Part model, mm, in its own coordinate system. A direction names the side the tool comes from. Give positions to 0.01 mm unless a question says otherwise; leave off trailing zeros. Loops run counter-clockwise (first coordinate to the right, second up) from the corner with the lowest first, then second, coordinate; pieces in that order, holes last. Notation, with made-up numbers: M -17.5,58.25 L 31.5,58.25 A15 cw 31.5,68.25 Z; hole C -33,-24.75 d2. An arc over 180 degrees is marked long. Put each result on its own line as item: value. Start each with the question number.
Autodesk Inventor part; units mm, degrees
ref_plane "YZ Plane" through (0, 0, 0) normal (1, 0, 0) x (0, 1, 0)
ref_plane "XZ Plane" through (0, 0, 0) normal (0, 1, 0) x (-1, 0, 0)
ref_plane "XY Plane" through (0, 0, 0) normal (0, 0, 1) x (1, 0, 0)
sketch "Sketch1" plane through (0, 0, 0) normal (0, 0, 1) x (1, 0, 0)
  line L0 (-28.08, -48.025) -> (28.08, -48.025)
  line L1 (28.08, -48.025) -> (28.08, 48.025)
  line L2 (28.08, 48.025) -> (-28.08, 48.025)
  line L3 (-28.08, 48.025) -> (-28.08, -48.025)
  line L4 (-28.08, -48.025) -> (28.08, 48.025) construction
  line L5 (28.08, -48.025) -> (-28.08, 48.025) construction
  point P0 (0, 0)
  dimension "Length" = 56.16
  dimension "Height" = 96.05
extrude "BasicShape" add sketch "Sketch1" along normal blind 5
sketch "KeypadDimensions" plane through (0, 0, 5) normal (0, 0, 1) x (1, 0, 0)
  line L0 (-28.08, -48.025) -> (28.08, -48.025) construction
  line L1 (28.08, -48.025) -> (3.93, -48.025) construction
  line L2 (3.93, -48.025) -> (3.93, 0) construction
  line L3 (3.93, 0) -> (28.08, 0) construction
  line L4 (28.08, 0) -> (28.08, -48.025) construction
  line L5 (-20.22, -40.2) -> (28.08, -40.2)
  line L6 (28.08, -40.2) -> (28.08, 40.2)
  line L7 (28.08, 40.2) -> (-20.22, 40.2)
  line L8 (-20.22, 40.2) -> (-20.22, -40.2)
  line L9 (-20.22, -40.2) -> (28.08, 40.2) construction
  line L10 (28.08, -40.2) -> (-20.22, 40.2) construction
  point P0 (0, 0)
  dimension "d4" = 24.15
  dimension "d5" = 48.025
  dimension "KeypadLength" = 48.3
  dimension "KeypadHeight" = 80.4
extrude "KeypadCountersink" cut sketch "KeypadDimensions" against normal blind 2
sketch "Sketch3" plane through (0, 0, 3) normal (0, 0, 1) x (1, 0, 0)
  line L0 (-20.22, -40.2) -> (-20.22, 40.2)
  line L1 (-20.22, 40.2) -> (-11.72, 40.2)
  line L2 (-11.72, 40.2) -> (-11.72, 31.7)
  line L3 (-11.72, 31.7) -> (-20.22, 31.7)
  line L4 (-20.22, 31.7) -> (-20.22, 40.2)
  line L5 (-20.22, 40.2) -> (28.08, 40.2)
  line L6 (28.08, 40.2) -> (19.58, 40.2)
  line L7 (19.58, 40.2) -> (19.58, 31.7)
  line L8 (19.58, 31.7) -> (28.08, 31.7)
  line L9 (28.08, 31.7) -> (28.08, 40.2)
  line L10 (28.08, -40.2) -> (-20.22, -40.2)
  line L11 (-20.22, -40.2) -> (-11.72, -40.2)
  line L12 (-11.72, -40.2) -> (-11.72, -31.7)
  line L13 (-11.72, -31.7) -> (-20.22, -31.7)
  line L14 (-20.22, -31.7) -> (-20.22, -40.2)
  line L15 (28.08, -40.2) -> (19.58, -40.2)
  line L16 (19.58, -40.2) -> (19.58, -31.7)
  line L17 (19.58, -31.7) -> (28.08, -31.7)
  line L18 (28.08, -31.7) -> (28.08, -40.2)
  line L19 (-11.72, 31.7) -> (19.58, 31.7)
  line L20 (-20.22, 40.2) -> (-16.27, 40.2) construction
  line L21 (-16.27, 40.2) -> (-16.27, 35.95) construction
  line L22 (-16.27, 35.95) -> (-20.22, 35.95) construction
  line L23 (-20.22, 35.95) -> (-20.22, 40.2) construction
  circle A0 centre (-16.27, 35.95) radius 1.75 construction
  circle A1 centre (-16.27, 35.95) radius 1.5
  line L24 (28.08, 40.2) -> (28.08, -40.2) construction
  line L25 (28.08, 40.2) -> (23.13, 40.2) construction
  line L26 (23.13, 40.2) -> (23.13, 35.95) construction
  line L27 (23.13, 35.95) -> (28.08, 35.95) construction
  line L28 (28.08, 35.95) -> (28.08, 40.2) construction
  circle A2 centre (23.13, 35.95) radius 1.5
  line L29 (28.08, -40.2) -> (23.13, -40.2) construction
  line L30 (23.13, -40.2) -> (23.13, -36.25) construction
  line L31 (23.13, -36.25) -> (28.08, -36.25) construction
  line L32 (28.08, -36.25) -> (28.08, -40.2) construction
  line L33 (-20.22, -40.2) -> (-16.27, -40.2) construction
  line L34 (-16.27, -40.2) -> (-16.27, -36.25) construction
  line L35 (-16.27, -36.25) -> (-20.22, -36.25) construction
  line L36 (-20.22, -36.25) -> (-20.22, -40.2) construction
  circle A3 centre (-16.27, -36.25) radius 1.5
  circle A4 centre (23.13, -36.25) radius 1.5
  point P0 (0, 0)
  dimension "d10" = 8.5
  dimension "d11" = 8.5
  dimension "d12" = 8.5
  dimension "d13" = 8.5
  dimension "CornerLength" = 8.5
  dimension "d15" = 8.5
  dimension "d16" = 8.5
  dimension "d17" = 8.5
  dimension "KeypadHoleDiameter" = 3.5
  dimension "KeypadScrewHoleDiameterUntapped" = 3
  dimension "UpperKeypadHoleSpacingY" = 4.25
  dimension "LeftKeypadHoleSpacingX" = 3.95
  dimension "RightKeypadHoleSpacingX" = 4.95
  dimension "d23" = 4.25
  dimension "d25" = 3
  dimension "d26" = 4.95
  dimension "LowerKeypadHoleSpacingY" = 3.95
  dimension "d28" = 3
  dimension "d29" = 3
  dimension "d30" = 3.95
  dimension "d31" = 3.95
extrude "Extrusion3" cut sketch "Sketch3" against normal blind 5 contours L2 L5 L7 L19 | A1 | A2 | A3 | A4
thread "Thread1"
thread "Thread2"
thread "Thread3"
thread "Thread4"
equation "\"d4\" = 0.5 * KeypadLength"
equation "\"d5\" = 0.5 * Height"
equation "\"d15\" = CornerLength"
equation "\"d16\" = CornerLength"
equation "\"d17\" = CornerLength"
equation "\"d23\" = UpperKeypadHoleSpacingY"
equation "\"d25\" = KeypadScrewHoleDiameterUntapped"
equation "\"d26\" = RightKeypadHoleSpacingX"
equation "\"d28\" = KeypadScrewHoleDiameterUntapped"
equation "\"d29\" = KeypadScrewHoleDiameterUntapped"
equation "\"d30\" = LowerKeypadHoleSpacingY"
equation "\"d31\" = LeftKeypadHoleSpacingX"
equation "\"d32\" = Thickness"
equation "\"d34\" = Thickness"
equation "\"d36\" = Thickness"
equation "\"d38\" = Thickness"
properties part number "2020-04-12 KeypadOnly"
1) Wall check: L1, parallel to Y at x = -16.27, z = 0.8 (3 decimals); L2, parallel to Y at x = 3, z = 0.5 (3 decimals); L3, parallel to Y at x = -3, z = 3.55 (3 decimals). Give the ranges that are in metal, low to high.
2) Band-saw the part on A-A on x = 17.5. Give the cut face in (y, z) (3 decimals), then the cut area to 3 significant figures.
3) Pin check, flat tip, straight feed: pin 1 Ø5 at (x, y) = (23.13, -36.25) entering from +Z. Stop position of the tip, or through.
4) Band-saw the part on D-D on z = 0.95. Give the cut face in (x, y) (3 decimals), then the cut area to 3 significant figures.
5) Band-saw the part on B-B on y = 35.95. Give the cut face in (x, z), then the cut area to 3 significant figures.
6) Mould opens along X. For faces 1 (the flat face through (4, -40.2, 4)), 2 (the flat face through (-11.72, 36, 2)), 3 (the flat face through (-28.08, 1, 2)) say: +X half, -X half, draft (parallel to the pull), parting line (faces both ways), or undercut.
7) Which spindle directions (+Z, -Z, +X, -X, +Y, -Y) get a long thin tool onto all of the face, cutting with end or side? Do faces 4 (the flat face through (19.58, 36, 2)), 5 (the flat face through (4, 40.2, 3)), 6 (the flat face through (4, 1, 3)). Say none if no direction does.
8) Band-saw the part on C-C on x = -16.27. Give the cut face in (y, z) (3 decimals).
Evaluation:
1. L1: -48.025 to -37.75, -34.75 to 34.45, 37.45 to 48.025
1. L2: -48.025 to 31.7, 40.2 to 48.025
1. L3: -48.025 to -40.2, 40.2 to 48.025
2. outline: M -48.025,0 L 31.7,0 L 31.7,3 L -40.2,3 L -40.2,5 L -48.025,5 Z; M 40.2,0 L 48.025,0 L 48.025,5 L 40.2,5 Z
2. area: 294 mm2
3. pin 1: z = 3
4. outline: M -28.08,-48.025 L 28.08,-48.025 L 28.08,48.025 L -28.08,48.025 Z; hole C -16.27,-36.25 d3; hole C -16.27,35.95 d3; hole M -11.72,31.7 L 19.58,31.7 L 19.58,40.2 L -11.72,40.2 Z; hole C 23.13,-36.25 d3; hole C 23.13,35.95 d3
4. area: 5,100 mm2
5. outline: M -28.08,0 L -17.77,0 L -17.77,3 L -20.22,3 L -20.22,5 L -28.08,5 Z; M -14.77,0 L -11.72,0 L -11.72,3 L -14.77,3 Z; M 19.58,0 L 21.63,0 L 21.63,3 L 19.58,3 Z; M 24.63,0 L 28.08,0 L 28.08,3 L 24.63,3 Z
5. area: 72.3 mm2
6. face 1: draft
6. face 2: undercut
6. face 3: -X half
7. face 4: +Z, -Z
7. face 5: +Z
7. face 6: +Z, +X
8. outline: M -48.025,0 L -37.75,0 L -37.75,3 L -40.2,3 L -40.2,5 L -48.025,5 Z; M -34.75,0 L 34.45,0 L 34.45,3 L -34.75,3 Z; M 37.45,0 L 48.025,0 L 48.025,5 L 40.2,5 L 40.2,3 L 37.45,3 Z
